```python
from build123d import *

# Parameters (mm, degrees)
SKETCH2_R           = 3
SKETCH2_R_2         = 8.5
SKETCH2_R_3         = 1.5
BOSS_EXTRUDE1_DEPTH = 5
SKETCH3_W           = 5
SKETCH3_H           = 31
BOSS_EXTRUDE2_DEPTH = 10
SKETCH4_R           = 1.5
SKETCH4_W           = 5
SKETCH4_H           = 20
CUT_EXTRUDE1_DEPTH  = 10


with BuildPart() as part:
    # Sketch2 → Boss-Extrude1 (new body)
    with BuildSketch(Plane.XY):
        Polygon((0, 0), (10, 0), (10, -5), (30, -5), (30, 0), (50, 0), (50, -5), (70, -5), (70, 0), (80, 0), (80, 5), (75, 5), (75, 23), (75, 25), (80, 25), (80, 31), (70, 31), (70, 36), (50, 36), (50, 31), (0, 31), align=None)
        with Locations((21, 14.5)):
            Circle(SKETCH2_R, mode=Mode.SUBTRACT)
        with Locations((41, 14.5)):
            Circle(SKETCH2_R_2, mode=Mode.SUBTRACT)
        with Locations((61, 14.5)):
            Circle(SKETCH2_R_2, mode=Mode.SUBTRACT)
        with Locations((30, 23.5)):
            Circle(SKETCH2_R_3, mode=Mode.SUBTRACT)
        with Locations((30, 5.5)):
            Circle(SKETCH2_R_3, mode=Mode.SUBTRACT)
    extrude(amount=-BOSS_EXTRUDE1_DEPTH)

    # Sketch3 → Boss-Extrude2 (add)
    with BuildSketch(Plane.ZY):
        with Locations((-2.5, 15.5)):
            Rectangle(SKETCH3_W, SKETCH3_H)
    extrude(amount=BOSS_EXTRUDE2_DEPTH)

    # Sketch4 → Cut-Extrude1 (cut)
    with BuildSketch(Plane.XY):
        with Locations((-3, 23.5)):
            Circle(SKETCH4_R)
        with Locations((-3, 5.5)):
            Circle(SKETCH4_R)
        with Locations((2.5, 15)):
            Rectangle(SKETCH4_W, SKETCH4_H)
    extrude(amount=-CUT_EXTRUDE1_DEPTH, mode=Mode.SUBTRACT)


solid = part.part
```
Check sheet for the modelled part. Datum: model origin and axes. Units: mm. A direction names the side the tool comes from. Coordinates: 2 decimals unless noted, no trailing zeros. Order: outer loops, then holes, each group sorted by start corner. A loop starts at its lowest first (then second) coordinate and runs counter-clockwise, first axis right, second up. Notation, with made-up numbers: (-27.75, -34) -> (11.25, -34) arc R8 ccw to (11.25, -25) -> close; hole circle Ø8 at (79, 85). An arc over 180 degrees is marked (long way). Write item = value, one per line. Start each with the question number.
1) Go/stop test with flat-tipped pins: P1, Ø2.5, axis at x = 30, y = 23.5, coming from the +Z side; P2, Ø2.5, axis at x = 3, z = -2.5, coming from the -Y side; P3, Ø1.5, axis at x = 74.5, z = -2.5, coming from the +Y side. Record where each tip stops, or that it passes through.
2) Material ranges on L1, parallel to Y at x = -3, z = -1.7; L2, parallel to Y at x = 4.5, z = -1.7; L3, parallel to Y at x = 41, z = -1.75, recorded low to high.
3) Access from +Z, -Z, +X, -X, +Y, -Y to the whole of each face (thin tool, end or side, straight path). Record for faces 1 (the flat face through (75, 15, -2)), 2 (the flat face through (2, 5, -2)), 3 (the flat face through (30, -3, -2)), 4 (the flat face through (75, 0, -2)).
4) Mould release check, pull along X, two halves, no side actions. Record for faces 5 (the flat face through (5, 15, -2)), 6 (the flat face through (50, 34, -2)), 7 (the flat face through (70, 33, -2)): +X half, -X half, draft (parallel to the pull), parting line (faces both ways), or undercut.
5) Cross-section at B-B (y = 14.5). Enter the section's corners in (x, z).
6) Cross-section at D-D (x = -3). Enter the section's corners in (y, z).
7) Cross-section at C-C (z = -2.95). State how many separate pieces and enclosed holes the cut face has, then the cut area to 3 significant figures.
8) Cross-section at A-A (x = 61). Enter the section's corners in (y, z).
Ans:
q1.P1 = through
q1.P2 = 0
q1.P3 = 31
q2.L1 = 0 to 4, 7 to 22, 25 to 31
q2.L2 = 0 to 5, 25 to 31
q2.L3 = 0 to 6, 23 to 31
q3.face_1 = +Z, -Z, +X
q3.face_2 = +Z, -Z
q3.face_3 = +Z, -Z, -Y
q3.face_4 = +Z, -Z, +X, -Y
q4.face_5 = undercut
q4.face_6 = -X half
q4.face_7 = +X half
q5.outline = (-10, -5) -> (0, -5) -> (0, 0) -> (-10, 0) -> close; (5, -5) -> (18, -5) -> (18, 0) -> (5, 0) -> close; (24, -5) -> (32.5, -5) -> (32.5, 0) -> (24, 0) -> close; (49.5, -5) -> (52.5, -5) -> (52.5, 0) -> (49.5, 0) -> close; (69.5, -5) -> (75, -5) -> (75, 0) -> (69.5, 0) -> close
q6.outline = (0, -5) -> (4, -5) -> (4, 0) -> (0, 0) -> close; (7, -5) -> (22, -5) -> (22, 0) -> (7, 0) -> close; (25, -5) -> (31, -5) -> (31, 0) -> (25, 0) -> close
q7.separate_pieces = 1
q7.enclosed_holes = 8
q7.area = 2,380 mm²
q8.outline = (-5, -5) -> (6, -5) -> (6, 0) -> (-5, 0) -> close; (23, -5) -> (36, -5) -> (36, 0) -> (23, 0) -> close
